Could you check a few things on this model? Use its own coordinates, in mm. A direction names the side the tool comes from. Coordinates: 2 decimals unless noted, no trailing zeros. Order: outer loops, then holes, each group sorted by start corner. A loop starts at its lowest first (then second) coordinate and runs counter-clockwise, first axis right, second up. Notation, with made-up numbers: (-13.75, 22.5) - (14.25, 22.5) arc R27 cw to (14.25, 46.5) - close; hole circle Ø8 at (76.5, 19). An arc over 180 degrees is marked (long way). One line per item, written item: value. Start each with the question number.
from build123d import *

# Parameters (mm, degrees)
SKETCH_1_W           = 94
SKETCH_1_H           = 26
SKETCH_1_R           = 1
EXTRUDE_1_DEPTH      = 3.5
SKETCH_2_W           = 4.7
SKETCH_2_H           = 8.9
SKETCH_2_W_2         = 59.6
SKETCH_2_H_2         = 6.6
CUT_EXTRUDE_1_DEPTH  = 49.890183064
SKETCH_3_R           = 1.5
CUT_EXTRUDE_2_DEPTH  = 49.890183064
SKETCH_4_R           = 1.75
CUT_EXTRUDE_3_DEPTH  = 2
SKETCH_5_W           = 7.8
SKETCH_5_H           = 2.6
SKETCH_5_W_2         = 8.6
SKETCH_5_H_2         = 2
CUT_EXTRUDE_4_DEPTH  = 6
SKETCH_5_3_W         = 15.6
SKETCH_5_3_H         = 2
CUT_EXTRUDE_5_DEPTH  = 20
SKETCH_6_W           = 70
SKETCH_6_H           = 19.6
SKETCH_6_W_2         = 18.8
SKETCH_6_H_2         = 3
SKETCH_6_W_3         = 82.8
SKETCH_6_H_3         = 11
SKETCH_6_W_4         = 3.2
SKETCH_6_H_4         = 5.2
CUT_EXTRUDE_12_DEPTH = 2
SKETCH_7_W           = 6.7
SKETCH_7_H           = 7.7
CUT_EXTRUDE_13_DEPTH = 0.5


with BuildPart() as part:
    # 草图1 → 凸台-拉伸1 (new body)
    with BuildSketch(Plane(origin=(0, 0, 0), x_dir=(1, 0, 0), z_dir=(0, 1, 0))):
        Rectangle(SKETCH_1_W, SKETCH_1_H)
        with Locations(Location((-44, 10, 0), (0, 0, 270))):
            Circle(SKETCH_1_R, mode=Mode.SUBTRACT)
        with Locations(Location((-44, -10, 0), (0, 0, 270))):
            Circle(SKETCH_1_R, mode=Mode.SUBTRACT)
        with Locations(Location((44, 10, 0), (0, 0, 270))):
            Circle(SKETCH_1_R, mode=Mode.SUBTRACT)
        with Locations(Location((44, -10, 0), (0, 0, 270))):
            Circle(SKETCH_1_R, mode=Mode.SUBTRACT)
    extrude(amount=EXTRUDE_1_DEPTH)

    # 草图2 → 切除-拉伸1 (cut, through all)
    with BuildSketch(Plane.XZ):
        with Locations((-44.65, 2.65)):
            Rectangle(SKETCH_2_W, SKETCH_2_H)
        with Locations((-4.8, 0)):
            Rectangle(SKETCH_2_W_2, SKETCH_2_H_2)
    extrude(amount=-CUT_EXTRUDE_1_DEPTH, mode=Mode.SUBTRACT)

    # 草图3 → 切除-拉伸2 (cut, through all)
    with BuildSketch(Plane(origin=(0, 0, 0), x_dir=(-1, 0, 0), z_dir=(0, -1, 0))):
        with Locations(Location((27.5, -10, 0), (0, 0, 90))):
            Circle(SKETCH_3_R)
    extrude(amount=-CUT_EXTRUDE_2_DEPTH, mode=Mode.SUBTRACT)

    # 草图4 → 切除-拉伸3 (cut)
    with BuildSketch(Plane.XZ):
        with Locations(Location((-44, 10, 0), (0, 0, 270))):
            Circle(SKETCH_4_R)
        with Locations(Location((-44, -10, 0), (0, 0, 270))):
            Circle(SKETCH_4_R)
        with Locations(Location((44, 10, 0), (0, 0, 270))):
            Circle(SKETCH_4_R)
        with Locations(Location((44, -10, 0), (0, 0, 270))):
            Circle(SKETCH_4_R)
    extrude(amount=-CUT_EXTRUDE_3_DEPTH, mode=Mode.SUBTRACT)

    # 草图5 → 切除-拉伸4 (cut)
    with BuildSketch(Plane.XY.offset(13)):
        with Locations((-37.2, 2.2)):
            Rectangle(SKETCH_5_W, SKETCH_5_H)
        with Locations((-27.5, 2.5)):
            Rectangle(SKETCH_5_W_2, SKETCH_5_H_2)
    extrude(amount=-CUT_EXTRUDE_4_DEPTH, mode=Mode.SUBTRACT)

    # 草图5<3> → 切除-拉伸5 (cut)
    with BuildSketch(Plane.XY.offset(13)):
        with Locations((32.9, 2.5)):
            Rectangle(SKETCH_5_3_W, SKETCH_5_3_H)
    extrude(amount=-CUT_EXTRUDE_5_DEPTH, mode=Mode.SUBTRACT)

    # 草图6 → 切除-拉伸12 (cut)
    with BuildSketch(Plane(origin=(0, 3.5, 0), x_dir=(1, 0, 0), z_dir=(0, 1, 0))):
        with Locations((-7.8, 2.7)):
            Rectangle(SKETCH_6_W, SKETCH_6_H)
        with Locations((36.6, 0)):
            Rectangle(SKETCH_6_W_2, SKETCH_6_H_2)
        with Locations((0.3, -7)):
            Rectangle(SKETCH_6_W_3, SKETCH_6_H_3)
        with Locations((-44.4, 5.4)):
            Rectangle(SKETCH_6_W_4, SKETCH_6_H_4)
    extrude(amount=-CUT_EXTRUDE_12_DEPTH, mode=Mode.SUBTRACT)

    # 草图7 → 切除-拉伸13 (cut)
    with BuildSketch(Plane(origin=(0, 1.5, 0), x_dir=(1, 0, 0), z_dir=(0, 1, 0))):
        with Locations((-27.35, 7.15)):
            Rectangle(SKETCH_7_W, SKETCH_7_H)
    extrude(amount=-CUT_EXTRUDE_13_DEPTH, mode=Mode.SUBTRACT)


solid = part.part
Q1. We'd pull the mould along X, two halves only. Please class faces 1 (the flat face through (-42.3, 1, 3)), 2 (the flat face through (43, 2, 9)), 3 (the flat face through (-44, 2, 7.1)): +X half, -X half, draft (parallel to the pull), parting line (faces both ways), or undercut.
Q2. I want a section at C-C on x = -27.5. Please give me the cut outline in (y, z).
Q3. I'm going to push flat-ended pins straight in: pin 1 (3 mm diameter, centred on x = 31, z = 9.5, fed in from +Y); pin 2 (1.6 mm diameter, centred on x = -44, z = -10, fed in from -Y); pin 3 (3 mm diameter, centred on x = -44, z = -10, fed in from -Y). Where does each tip first touch, or does it pass through?
Q4. I want a section at B-B on z = 10. State how many separate pieces and enclosed holes the cut face has, then the cut area to 3 significant figures.
Q5. I want a section at A-A on x = 9.5. Please give me the cut outline in (y, z).
Q6. Which directions (+Z, -Z, +X, -X, +Y, -Y) give clear straight access to the entire face, cutting with the end or side of a thin tool? Please do faces 4 (the flat face through (1, 3, 12.5)), 5 (the flat face through (43, 3, -1.5)), 6 (the cylindrical face through (42.29, 0.99, -9.62)).
Q7. If I drill on L1, parallel to X at y = 2.55, z = -10; L2, parallel to X at y = 0.5, z = -10; L3, parallel to Z at x = -44, y = 3.25, over which ranges is the centre line in solid material (lowest first)?
Q8. I want a section at D-D on z = 0.5. Please give me the cut outline in (x, y).
Values follow:
1. face 1: -X half
1. face 2: undercut
1. face 3: draft
2. outline: (0, -13) - (3.5, -13) - (3.5, -12.5) - (1.5, -12.5) - (1.5, -11) - (1, -11) - (1, -3.3) - (0, -3.3) - close; (0, 3.3) - (1.5, 3.3) - (1.5, 8.5) - (0, 8.5) - close; (0, 11.5) - (1.5, 11.5) - (1.5, 13) - (0, 13) - close
3. pin 1: stops at y = 1.5
3. pin 2: passes through
3. pin 3: stops at y = 2
4. separate pieces: 4
4. enclosed holes: 0
4. area: 134 mm^2
5. outline: (0, -13) - (3.5, -13) - (3.5, -12.5) - (1.5, -12.5) - (1.5, -3.3) - (0, -3.3) - close; (0, 3.3) - (1.5, 3.3) - (1.5, 12.5) - (3.5, 12.5) - (3.5, 13) - (0, 13) - close
6. face 4: +Y
6. face 5: -X, +Y
6. face 6: -Y
7. L1: x = -47 to -45, -43 to -42.8, 27.2 to 43, 45 to 47
7. L2: x = -47 to -45.75, -42.25 to 42.25, 45.75 to 47
7. L3: z = -13 to -11, -9 to -8, -2.8 to -1.8, 7.1 to 9, 11 to 13
8. outline: (-42.3, 0) - (-34.6, 0) - (-34.6, 1.5) - (-42.3, 1.5) - close; (25, 0) - (47, 0) - (47, 3.5) - (46, 3.5) - (46, 1.5) - (25, 1.5) - close
